Can you work these out from the model? Positions are in its coordinate system, mm. Face numbers are marked on the shaded views. A direction names the side the tool comes from. Give positions to 0.01 mm unless a question says otherwise; leave off trailing zeros. Loops run counter-clockwise (first coordinate to the right, second up) from the corner with the lowest first, then second, coordinate; pieces in that order, holes last. Notation, with made-up numbers: M 61.25,-5 L 98.25,-5 A25 ccw 98.25,14 Z; hole C 26.25,-26 d4. An arc over 180 degrees is marked long. Put each result on its own line as item: value. Start each with the question number.
1) Imagine slicing it at A-A (z = 0). Write out the boundary of the cut face in (x, y), then the cut area to 3 significant figures.
2) For P1, Ø1, axis at x = -45, y = -0.5, coming from the -Z side; P2, Ø4, axis at x = -18.5, y = 2, coming from the +Z side; P3, Ø1, axis at x = 12, z = 2, coming from the -Y side, each with a flat end and sliding along its axis, tell me the tip position at first contact or that it passes through.
3) Imagine slicing it at C-C (x = 52). Write out the boundary of the cut face in (y, z).
4) Please list where these lines run through material, in increasing order: line 1 along X through (y, z) = (0, -4.5); line 2 along Y through (x, z) = (15, 0); line 3 along Z through (x, y) = (19, 0.25). Write a range as from..to.
5) For the marked faces 1 and 2, which set-ups out of +Z, -Z, +X, -X, +Y, -Y let a thin tool reach every point of the face, with its end or its side?
6) Imagine slicing it at D-D (z = -5). Write out the boundary of the cut face in (x, y).
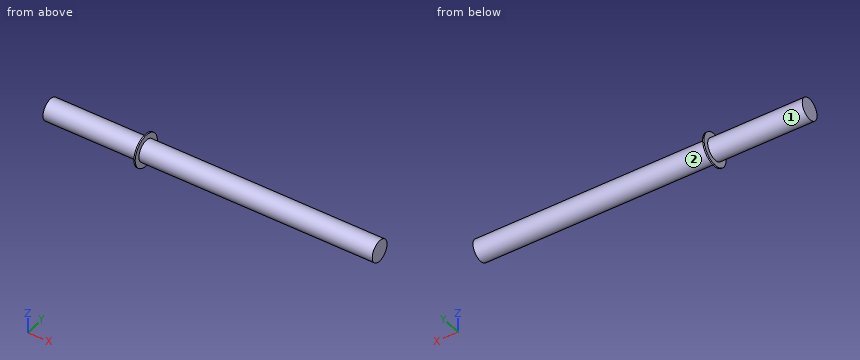
from build123d import *

# Parameters (mm, degrees)
ESBO_O1_W = 121.7
ESBO_O1_H = 4
ESBO_O2_W = 0.5
ESBO_O2_H = 6


with BuildPart() as part:
    # Esboço1 → Revolução2 (revolve)
    with BuildSketch(Plane.XY, mode=Mode.PRIVATE) as revolu_o2_sk:
        with Locations((0, -2)):
            Rectangle(ESBO_O1_W, ESBO_O1_H)
    revolve(revolu_o2_sk.sketch.rotate(Axis((-60.85, 0, 0), (1, 0, 0)), 270), axis=Axis((-60.85, 0, 0), (1, 0, 0)))

    # Esboço2 → Revolução3 (revolve)
    with BuildSketch(Plane.XY, mode=Mode.PRIVATE) as revolu_o3_sk:
        with Locations((-25.65, -3)):
            Rectangle(ESBO_O2_W, ESBO_O2_H)
    revolve(revolu_o3_sk.sketch.rotate(Axis((-25.9, 0, 0), (1, 0, 0)), 270), axis=Axis((-25.9, 0, 0), (1, 0, 0)))


solid = part.part
Recorded:
1. outline: M -60.85,-4 L -25.9,-4 L -25.9,-6 L -25.4,-6 L -25.4,-4 L 60.85,-4 L 60.85,4 L -25.4,4 L -25.4,6 L -25.9,6 L -25.9,4 L -60.85,4 Z
1. area: 976 mm²
2. P1: z = -4
2. P2: z = 4
2. P3: y = -3.71
3. outline: C 0,0 d8
4. line 1: -25.9..-25.4
4. line 2: -4..4
4. line 3: -3.99..3.99
5. face 1: -X
5. face 2: +X
6. outline: M -25.9,-3.32 L -25.4,-3.32 L -25.4,3.32 L -25.9,3.32 Z
